Can you work these out from the model? Positions are in its coordinate system, mm. A direction names the side the tool comes from. Round coordinates to 2 decimals unless told otherwise and drop trailing zeros. Order: outer loops, then holes, each group sorted by start corner. A loop starts at its lowest first (then second) coordinate and runs counter-clockwise, first axis right, second up. Notation, with made-up numbers: (69.5, 6.25) -> (75.5, 6.25) arc R23 cw to (75.5, 25.25) -> close; hole circle Ø1 at (-26.5, 55). An arc over 180 degrees is marked (long way). One line per item, written item: value.
```python
from build123d import *

# Parameters (mm, degrees)
SKETCH2_W           = 150
SKETCH2_H           = 150
BOSS_EXTRUDE1_DEPTH = 180
SKETCH5_R           = 30
BOSS_EXTRUDE3_DEPTH = 235
SKETCH7_R           = 50
CUT_EXTRUDE1_DEPTH  = 448.993409814


with BuildPart() as part:
    # Sketch2 → Boss-Extrude1 (new body)
    with BuildSketch(Plane.XY):
        with Locations((22.391402768, 2.285802295)):
            Rectangle(SKETCH2_W, SKETCH2_H)
    boss_extrude1 = extrude(amount=BOSS_EXTRUDE1_DEPTH)

    # Sketch5 → Boss-Extrude3 (add)
    with BuildSketch(Plane.XY.offset(180)):
        with Locations(Location((22.391402768, 2.285802295, 0), (0, 0, 180))):
            Circle(SKETCH5_R)
    boss_extrude3 = extrude(amount=BOSS_EXTRUDE3_DEPTH)

    # Mirror1: Boss-Extrude1, Boss-Extrude3 across plane
    add(boss_extrude1.mirror(Plane.XY))
    add(boss_extrude3.mirror(Plane.XY))

    # Sketch7 → Cut-Extrude1 (cut, through all)
    with BuildSketch(Plane(origin=(97.391402768, 0, 0), x_dir=(0, 0, -1), z_dir=(1, 0, 0))):
        with Locations((0, 2.285802295)):
            Circle(SKETCH7_R)
    extrude(amount=-CUT_EXTRUDE1_DEPTH, mode=Mode.SUBTRACT)


solid = part.part
```
Q1. Will these pins go through, and if not, where does the flat tip stop? pin 1 Ø8 at (x, y) = (58, 15) entering from -Z; pin 2 Ø4 at (x, y) = (30, -48) entering from +Z.
Answers below:
pin 1: z = -180
pin 2: z = 180
Q2. We'd pull the mould along Z, two halves only. Please class faces 3 (the face through (52.362, 0.967, -295.855)), 4 (the face through (-12, 3, 180)), 5 (the face through (-12, 3, -180)), 6 (the face through (23.44, -16.86, -46.19)): released by +Z, released by -Z, zero draft, split by the parting line, or undercut.
Answers below:
face 3: zero draft
face 4: released by +Z
face 5: released by -Z
face 6: undercut
Q3. On a 3-axis mill with a long thin cutter (end or side, diameter ignored), from which of +Z, -Z, +X, -X, +Y, -Y can I reach the whole of each face in a straight line? I mean faces 1 (the face through (52.362, 0.967, 295.855)), 2 (the face through (-52.609, -49, 3)). Say none if no direction works.
Answers below:
face 1: +Z
face 2: +Z, -Z, -X, +Y, -Y
Q4. I want a section at D-D on z = 275. List the corners of the cut face in (x, y) for me, plus the area to 3 significant figures.
Answers below:
outline: circle Ø60 at (22.39, 2.29)
area: 2,830 mm^2
Q5. I want a section at B-B on x = 17. List the corners of the cut face in (y, z) for me, plus the area to 3 significant figures.
Answers below:
outline: (-72.71, -180) -> (-27.23, -180) -> (-27.23, -415) -> (31.8, -415) -> (31.8, -180) -> (77.29, -180) -> (77.29, 180) -> (31.8, 180) -> (31.8, 415) -> (-27.23, 415) -> (-27.23, 180) -> (-72.71, 180) -> close; hole circle Ø100 at (2.29, 0)
area: 73,900 mm^2
Q6. I want a section at C-C on x = -18. List the corners of the cut face in (y, z) for me, plus the area to 3 significant figures.
Answers below:
outline: (-72.71, -180) -> (77.29, -180) -> (77.29, 180) -> (-72.71, 180) -> close; hole circle Ø100 at (2.29, 0)
area: 46,100 mm^2
Q7. Please list where these lines run through material, in increasing order: line 1 along Y through (x, z) = (-15, 0); line 2 along Z through (x, y) = (26, -5.5); line 3 along Z through (x, y) = (8, 14).
Answers below:
line 1: -72.71 to -47.71, 52.29 to 77.29
line 2: -415 to -49.39, 49.39 to 415
line 3: -415 to -48.61, 48.61 to 415
Q8. I want a section at A-A on z = 0. List the corners of the cut face in (x, y) for me.
Answers below:
outline: (-52.61, -72.71) -> (97.39, -72.71) -> (97.39, -47.71) -> (-52.61, -47.71) -> close; (-52.61, 52.29) -> (97.39, 52.29) -> (97.39, 77.29) -> (-52.61, 77.29) -> close
